Input: dimensioned drawing with shaded views. Units: mm. Origin: part minimum x, y, z. Give positions to 0.01 mm unless a question says otherwise; leave off trailing zeros. Write each loop counter-clockwise with the first axis right and the second up, starting at its lowest first coordinate (ties: lowest second). Pieces come first, ordered by that corner, then holes.
Q1. Section B-B (z = 12.5). Return the cut outline in (x, y).
Q2. Pin query (flat end, axial travel): pin 1 Ø1.8 at (x, y) = (51.5, 2.5) entering from +Z; pin 2 Ø1.6 at (x, y) = (16, 2.5) entering from +Z; pin 3 Ø3 at (x, y) = (59, 2.5) entering from -Z. Return the tip coordinate at first contact, or that it passes through.
Q3. Section C-C (z = 6.75). Return the cut outline in (x, y), plus the area to 3 significant figures.
Q4. Mould query, pull axis X, two halves, no side actions, for the marked faces 1 and 2. Classes: +X half, -X half, draft (parallel to the pull), parting line (faces both ways), or undercut.
Q5. Line query: line 1 (X direction, y = 2.5, z = 7.05); line 2 (Y direction, x = 16, z = 21.5); line 3 (X direction, y = 2.5, z = 8). Output: solid intervals per line, ascending.
Q6. Section A-A (x = 37.5). Return the cut outline in (y, z), plus the area to 3 significant figures.
Q7. Section D-D (x = 12). Return the cut outline in (y, z), plus the area to 3 significant figures.
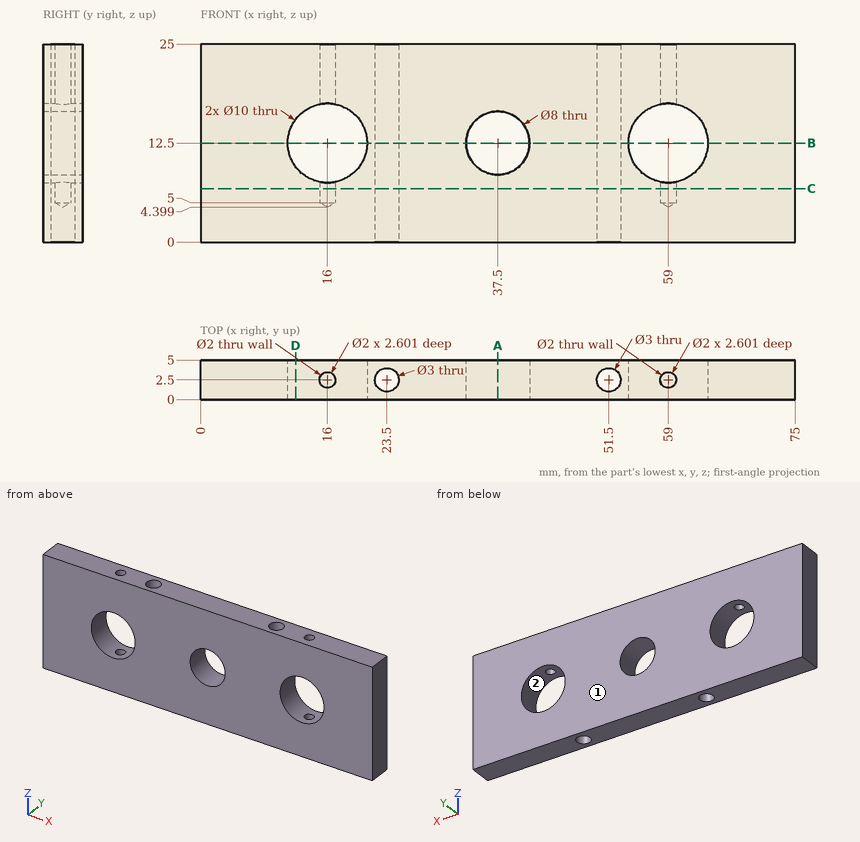
Computed:
1. outline: (0, 0) - (11, 0) - (11, 5) - (0, 5) - close; (21, 0) - (33.5, 0) - (33.5, 5) - (21, 5) - close; (41.5, 0) - (54, 0) - (54, 5) - (41.5, 5) - close; (64, 0) - (75, 0) - (75, 5) - (64, 5) - close; hole circle Ø3 at (23.5, 2.5); hole circle Ø3 at (51.5, 2.5)
2. pin 1: passes through
2. pin 2: stops at z = 4.88
2. pin 3: stops at z = 0
3. outline: (0, 0) - (75, 0) - (75, 5) - (0, 5) - close; hole circle Ø2 at (16, 2.5); hole circle Ø3 at (23.5, 2.5); hole circle Ø3 at (51.5, 2.5); hole circle Ø2 at (59, 2.5)
3. area: 355 mm2
4. face 1: draft
4. face 2: undercut
5. line 1: x = 0 to 15, 17 to 22, 25 to 50, 53 to 58, 60 to 75
5. line 2: y = 0 to 1.5, 3.5 to 5
5. line 3: x = 0 to 13.82, 18.18 to 22, 25 to 50, 53 to 56.82, 61.18 to 75
6. outline: (0, 0) - (5, 0) - (5, 8.5) - (0, 8.5) - close; (0, 16.5) - (5, 16.5) - (5, 25) - (0, 25) - close
6. area: 85.0 mm2
7. outline: (0, 0) - (5, 0) - (5, 9.5) - (0, 9.5) - close; (0, 15.5) - (5, 15.5) - (5, 25) - (0, 25) - close
7. area: 95.0 mm2
